Here's how the part is built. I have some questions about the finished solid (model axes, mm). A direction names the side the tool comes from. Round coordinates to 2 decimals unless told otherwise and drop trailing zeros. Loops run counter-clockwise (first coordinate to the right, second up) from the corner with the lowest first, then second, coordinate; pieces in that order, holes last. Notation, with made-up numbers: M 46.5,-14 L 72.5,-14 A24 cw 72.5,13 Z; hole C 10.25,41.25 d1. An arc over 180 degrees is marked long. Answer as a JSON object with one key per item and string values.
from build123d import *

# Parameters (mm, degrees)
SKETCH1_W           = 60
SKETCH1_H           = 50
BOSS_EXTRUDE2_DEPTH = 50
SKETCH2_W           = 10
SKETCH2_H           = 20
CUT_EXTRUDE1_DEPTH  = 50
SKETCH3_W           = 30
SKETCH3_H           = 20
CUT_EXTRUDE2_DEPTH  = 20
CUT_EXTRUDE4_DEPTH  = 40


with BuildPart() as part:
    # Sketch1 → Boss-Extrude2 (new body)
    with BuildSketch(Plane.XY):
        with Locations((30, 25)):
            Rectangle(SKETCH1_W, SKETCH1_H)
    extrude(amount=BOSS_EXTRUDE2_DEPTH)

    # Sketch2 → Cut-Extrude1 (cut)
    with BuildSketch(Plane.XY.offset(50)):
        with Locations((5, 40)):
            Rectangle(SKETCH2_W, SKETCH2_H)
    extrude(amount=-CUT_EXTRUDE1_DEPTH, mode=Mode.SUBTRACT)

    # Sketch3 → Cut-Extrude2 (cut)
    with BuildSketch(Plane.XY.offset(50)):
        with Locations((15, 10)):
            Rectangle(SKETCH3_W, SKETCH3_H)
    extrude(amount=-CUT_EXTRUDE2_DEPTH, mode=Mode.SUBTRACT)

    # Sketch4 → Cut-Extrude4 (cut)
    with BuildSketch(Plane.XY.offset(50)):
        Polygon((30, 20), (50, 50), (10, 50), (10, 30), (0, 30), (0, 20), align=None)
    extrude(amount=-CUT_EXTRUDE4_DEPTH, mode=Mode.SUBTRACT)


solid = part.part
Item 1: I want a section at B-B on y = 41. List the corners of the cut face in (x, z) for me, plus the area to 3 significant figures.
Solution:
{"outline": "M 10,0 L 60,0 L 60,50 L 44,50 L 44,10 L 10,10 Z", "area": "1,140 mm2"}
Item 2: For faces 1 (the face through (5, 30, 5)), 2 (the face through (36, 0, 19)), 3 (the face through (25, 35, 10)), 4 (the face through (30, 10, 40)), which set-ups out of +Z, -Z, +X, -X, +Y, -Y let a thin tool reach every point of the face, with its end or its side?
Solution:
{"face 1": "+Z, -Z, -X, +Y", "face 2": "+Z, -Z, +X, -X, -Y", "face 3": "+Z, -X, +Y", "face 4": "+Z, -X, +Y, -Y"}
Item 3: For P1, Ø2, axis at x = 10, y = 13, coming from the +Z side; P2, Ø11, axis at y = 37, z = 6, coming from the -X side; P3, Ø2, axis at y = 33, z = 26, coming from the -X side, each with a flat end and sliding along its axis, tell me the tip position at first contact or that it passes through.
Solution:
{"P1": "stops at z = 30", "P2": "stops at x = 10", "P3": "stops at x = 38"}
Item 4: I want a section at C-C on z = 33. List the corners of the cut face in (x, y) for me, plus the area to 3 significant figures.
Solution:
{"outline": "M 30,0 L 60,0 L 60,50 L 50,50 L 30,20 Z", "area": "1,200 mm2"}
Item 5: If I drill on L1, parallel to Z at x = 44.5, y = 45.5; L2, parallel to Z at x = 4, y = 19; L3, parallel to X at y = 10, z = 33.5, over which ranges is the centre line in solid material (lowest first)? Write a range as from..to.
Solution:
{"L1": "z = 0..10", "L2": "z = 0..30", "L3": "x = 30..60"}
Item 6: I want a section at A-A on x = 23. List the corners of the cut face in (y, z) for me, plus the area to 3 significant figures.
Solution:
{"outline": "M 0,0 L 50,0 L 50,10 L 20,10 L 20,30 L 0,30 Z", "area": "900 mm2"}
